The listing builds one solid part. Answer for the finished solid, in the listing's coordinates (mm). Face numbers are marked on the shaded views. Give positions to 0.01 mm unless a question says otherwise; leave off trailing zeros. Order: outer loops, then holes, each group sorted by start corner. A loop starts at its lowest first (then second) coordinate and runs counter-clockwise, first axis right, second up. Notation, with made-up numbers: (63.25, -40) - (67.25, -40) arc R11 ccw to (67.25, -32) - close; hole circle Ø7 at (87, 49.25). An arc over 180 degrees is marked (long way). Use a Markdown table: item, result. Add a question column.
1) Straight lines are drawn through the part: line 1 (X direction, y = 0, z = -1); line 2 (X direction, y = 0, z = -4); line 3 (Z direction, x = -21, y = 2.5). For each, find the intervals that lie inside material, in ascending order.
2) Find section C-C, the plane z = -26.5. Determine the outline of the cut face in (x, y).
3) Flat-ended cylindrical pins translate along their axes: pin 1 (17 mm diameter, centred on x = -4.5, y = 0.5, fed in from -Z); pin 2 (1 mm diameter, centred on x = 6, z = -19, fed in from +Y); pin 3 (2 mm diameter, centred on y = -14.5, z = -17, fed in from -X); pin 4 (6 mm diameter, centred on y = -5, z = -27.5, fed in from -X). Find the tip coordinate at first contact, or state that the pin passes through.
4) The mould has two halves that part along Y. Classify the marked faces 1, 2 and 3: released by +Y, released by -Y, zero draft, split by the parting line, or undercut.
Autodesk Inventor part; units mm, degrees
ref_plane "YZ Plane" through (0, 0, 0) normal (1, 0, 0) x (0, 1, 0)
ref_plane "XZ Plane" through (0, 0, 0) normal (0, 1, 0) x (-1, 0, 0)
ref_plane "XY Plane" through (0, 0, 0) normal (0, 0, 1) x (1, 0, 0)
sketch "Sketch2" plane through (0, 0, 0) normal (1, 0, 0) x (0, 1, 0)
  line L0 (17.05, -2) -> (17.05, -10)
  line L1 (17.05, -10) -> (21.6, -10)
  line L2 (21.6, -10) -> (21.6, -46)
  line L3 (21.6, -46) -> (24, -46)
  line L4 (24, -46) -> (24, -15)
  line L5 (24, -15) -> (25.4, -15)
  line L6 (25.4, -15) -> (25.4, 0)
  line L7 (25.4, 0) -> (17.05, 0)
  line L8 (0, 0) -> (0, -55.6888)
  line L9 (17.05, 0) -> (16.15, 0)
  line L10 (16.15, 0) -> (16.15, -2)
  line L11 (16.15, -2) -> (17.05, -2)
  line L12 (17.05, -2) -> (17.05, 0)
  point P0 (24.7, -15)
  dimension "d0" = 10
  dimension "d1" = 36
  dimension "d2" = 17.05
  dimension "d3" = 21.6
  dimension "d4" = 25.4
  dimension "d5" = 24
  dimension "d6" = 15
  dimension "d7" = 2
  dimension "d8" = 0.9
revolve "Revolution2" add sketch "Sketch2" angle 360 about axis through (0, 0, 0) along (0, 0, -1)
chamfer "Chamfer1" distance 0.5 angle 45 5 edges at (0, -25.4, 0) (0, -25.4, -15) (0, -16.15, 0) (0, -24, -46) (0, -21.6, -46)
properties part number "Nikon50mm-barebone-mount"
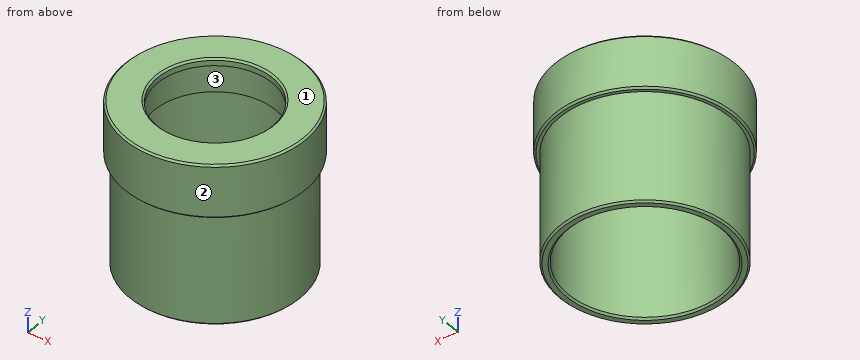
The answers:
| question | item | result |
|---|---|---|
| 1 | line 1 | -25.4 to -16.15, 16.15 to 25.4 |
| 1 | line 2 | -25.4 to -17.05, 17.05 to 25.4 |
| 1 | line 3 | -10 to 0 |
| 2 | outline | circle Ø48 at (0, 0); hole circle Ø43.2 at (0, 0) |
| 3 | pin 1 | through |
| 3 | pin 2 | y = 23.36 |
| 3 | pin 3 | x = -19.84 |
| 3 | pin 4 | x = -23.92 |
| 4 | face 1 | zero draft |
| 4 | face 2 | split by the parting line |
| 4 | face 3 | undercut |
